Answer from the drawing. Dimensions are ordinates in mm from the lowest x, y and z of the part. Round coordinates to 2 decimals unless told otherwise and drop trailing zeros. Loops run counter-clockwise (first coordinate to the right, second up) from the corner with the lowest first, then second, coordinate; pieces in that order, holes last. Notation, with made-up numbers: (20, 65) - (75, 65) arc R11 cw to (75, 69) - close; hole circle Ø5 at (-40, 8). An arc over 180 degrees is marked (long way). Write item = value, one per line. Start each with the question number.
1) Section A-A, the plane y = 139 is taken. Determine the outline of the cut face in (x, z) (1 decimal).
2) Section D-D, the plane x = 181 is taken. Determine the outline of the cut face in (y, z) (1 decimal).
3) Section B-B, the plane x = 68 is taken. Determine the outline of the cut face in (y, z) (1 decimal).
4) Given pin 1 Ø1.6 at (y, z) = (6, 2) entering from -X; pin 2 Ø1 at (x, z) = (104.5, 2) entering from +Y; pin 3 Ø1 at (y, z) = (24, 1.5) entering from +X, each flat-ended and moving along its own axis, determine where each tip first touches the part or whether it passes through.
5) Straight lines are drawn through the part: line 1 along Y through (x, z) = (33, 2.2) (1 decimal); line 2 along Y through (x, z) = (96.5, 0.75); line 3 along Y through (x, z) = (158, 1.35) (1 decimal). For each, find the intervals that lie inside material, in ascending order.
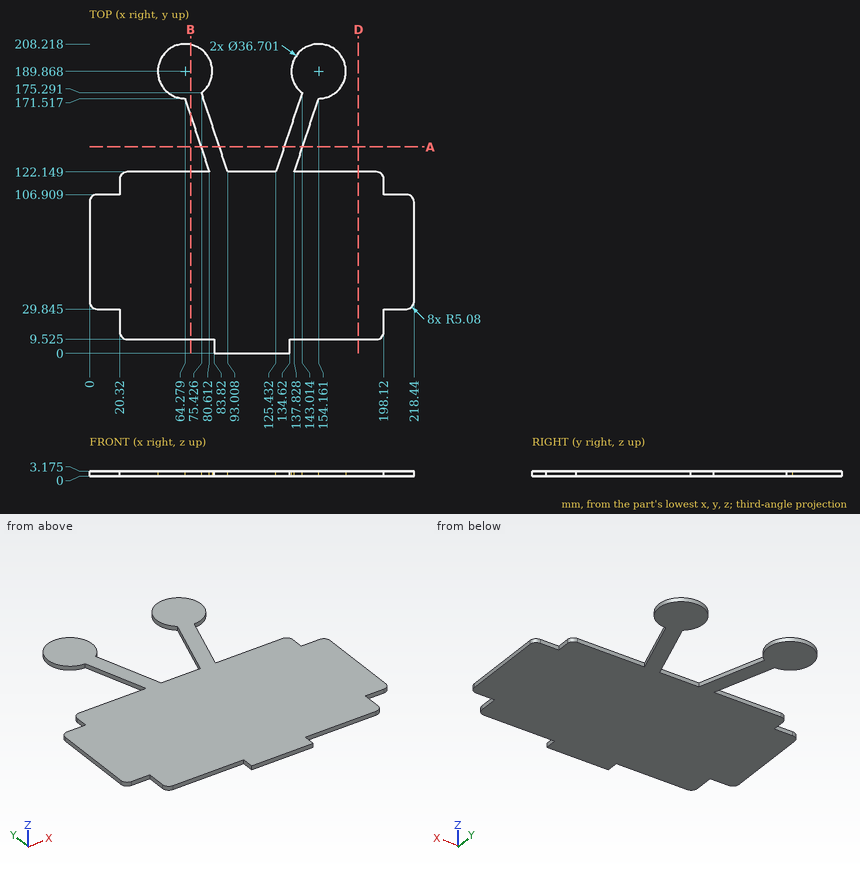
Geometry check:
q1.outline = (75, 0) - (87.4, 0) - (87.4, 3.2) - (75, 3.2) - close; (131, 0) - (143.4, 0) - (143.4, 3.2) - (131, 3.2) - close
q2.outline = (9.5, 0) - (122.1, 0) - (122.1, 3.2) - (9.5, 3.2) - close
q3.outline = (9.5, 0) - (122.1, 0) - (122.1, 3.2) - (9.5, 3.2) - close; (160.3, 0) - (207.8, 0) - (207.8, 3.2) - (160.3, 3.2) - close
q4.pin_1 = 83.82
q4.pin_2 = 122.15
q4.pin_3 = 198.12
q5.line_1 = 9.5 to 122.1
q5.line_2 = 0 to 122.15
q5.line_3 = 9.5 to 122.1, 171.9 to 207.8
